Geometry: final body of the model. Coordinates: model frame, mm. Face numbers are marked on the shaded views. A direction names the side the tool comes from. Round coordinates to 2 decimals unless told otherwise and drop trailing zeros. Write each loop counter-clockwise with the first axis right and the second up, starting at its lowest first coordinate (ties: lowest second). Pieces come first, ordered by that corner, then holes. Notation, with made-up numbers: (-21, 21.25) -> (7, 21.25) arc R11 cw to (7, 26.25) -> close; hole circle Ø1 at (66, 47.25). An arc over 180 degrees is marked (long way). Use one line per item in the form item = value. Start each with the question number.
1. Cut plane A-A, the plane z = 14. Return the cut outline in (x, y), plus the area to 3 significant figures.
2. Cut plane D-D, the plane z = 25. Return the cut outline in (x, y).
3. Cut plane B-B, the plane y = 0. Return the cut outline in (x, z) (3 decimals), plus the area to 4 significant figures.
4. Cut plane C-C, the plane x = 30. Return the cut outline in (y, z) (3 decimals).
5. Line query: L1, parallel to Y at x = 30, z = 30; L2, parallel to X at y = 0, z = 15; L3, parallel to X at y = 0, z = 22. Output: solid intervals per line, ascending.
6. Draft query along Y for the marked faces 3, 4 and 5. Return one class per face: pulls with the +Y half, pulls with the -Y half, needs draft (parallel to the pull), parting line crosses it, or undercut.
7. Pin query (flat end, axial travel): pin 1 Ø4 at (x, y) = (12.5, -43) entering from +Z; pin 2 Ø5 at (x, z) = (44.5, 34) entering from +Y. Return the tip coordinate at first contact, or that it passes through.
8. Reachability of the marked faces 1 and 2 from +Z, -Z, +X, -X, +Y, -Y: full face, straight path, thin tool, end or side. Return the list, or none.
```python
from build123d import *

# Parameters (mm, degrees)
F1_DEPTH = 60
F2_R     = 16
F3_DEPTH = 25
F4_R     = 20.225
F4_R_2   = 16
F5_DEPTH = 10
F6_R     = 24
F6_R_2   = 16
F7_DEPTH = 16


with BuildPart() as f1:
    # F0 (on Right) → F1 (new body)
    with BuildSketch(Plane.YZ):
        Polygon((-100, 31), (-100, 0), (-40, 0), (-40, 16), (0, 16), (40, 16), (40, 0), (100, 0), (100, 31), align=None)
    extrude(amount=F1_DEPTH)

    # F2 (on face) → F3 (cut)
    with BuildSketch(Plane.XY.offset(31)):
        with Locations((30, 0)):
            Circle(F2_R)
    extrude(amount=-F3_DEPTH, mode=Mode.SUBTRACT)

    # F4 (on face) → F5 (join)
    with BuildSketch(Plane.XY.offset(31)):
        with Locations((30, 0)):
            Circle(F4_R)
        with Locations((30, 0)):
            Circle(F4_R_2, mode=Mode.SUBTRACT)
    extrude(amount=F5_DEPTH)

    # F6 (on face) → F7 (join)
    with BuildSketch(Plane(origin=(0, 0, 16), x_dir=(1, 0, 0), z_dir=(0, 0, -1))):
        with Locations((30, 0)):
            Circle(F6_R)
        with Locations((30, 0)):
            Circle(F6_R_2, mode=Mode.SUBTRACT)
    extrude(amount=F7_DEPTH)


solid = f1.part
```
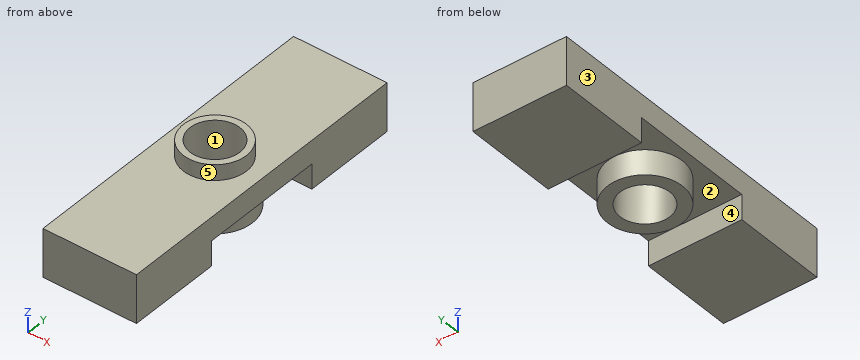
Outcome:
q1.outline = (0, -100) -> (60, -100) -> (60, -40) -> (0, -40) -> close; (0, 40) -> (60, 40) -> (60, 100) -> (0, 100) -> close; circle Ø48 at (30, 0); hole circle Ø32 at (30, 0)
q1.area = 8,210 mm^2
q2.outline = (0, -100) -> (60, -100) -> (60, 100) -> (0, 100) -> close; hole circle Ø32 at (30, 0)
q3.outline = (0, 16) -> (6, 16) -> (6, 0) -> (14, 0) -> (14, 41) -> (9.775, 41) -> (9.775, 31) -> (0, 31) -> close; (46, 0) -> (54, 0) -> (54, 16) -> (60, 16) -> (60, 31) -> (50.225, 31) -> (50.225, 41) -> (46, 41) -> close
q3.area = 760.5 mm^2
q4.outline = (-100, 0) -> (-40, 0) -> (-40, 16) -> (-24, 16) -> (-24, 0) -> (-16, 0) -> (-16, 41) -> (-20.225, 41) -> (-20.225, 31) -> (-100, 31) -> close; (16, 0) -> (24, 0) -> (24, 16) -> (40, 16) -> (40, 0) -> (100, 0) -> (100, 31) -> (20.225, 31) -> (20.225, 41) -> (16, 41) -> close
q5.L1 = -100 to -16, 16 to 100
q5.L2 = 6 to 14, 46 to 54
q5.L3 = 0 to 14, 46 to 60
q6.face_3 = needs draft
q6.face_4 = undercut
q6.face_5 = parting line crosses it
q7.pin_1 = 31
q7.pin_2 = 16.28
q8.face_1 = +Z, -Z
q8.face_2 = -Z
